Check sheet for the modelled part. Datum: model origin and axes. Units: mm. Face numbers are marked on the shaded views. A direction names the side the tool comes from. Round coordinates to 2 decimals unless told otherwise and drop trailing zeros. Write each loop counter-clockwise with the first axis right and the second up, starting at its lowest first coordinate (ties: lowest second). Pieces come first, ordered by that corner, then holes.
Item 1: Cross-section at A-A on y = -9.5. Enter the section's corners in (x, z), plus the area to 3 significant figures.
Item 2: Material ranges on line 1 (Z direction, x = -2, y = -8); line 2 (X direction, y = -3, z = 1); line 3 (Y direction, x = -6, z = 2.25), recorded low to high.
Item 3: Go/stop test with flat-tipped pins: pin 1 Ø3 at (x, y) = (0, -7) entering from +Z; pin 2 Ø1.2 at (y, z) = (-18.5, 0.5) entering from +X; pin 3 Ø2 at (y, z) = (13, 1.5) entering from -X. Record where each tip stops, or that it passes through.
Item 4: Tool access check on the marked faces 1, 2 and 3. Record the directions out of +Z, -Z, +X, -X, +Y, -Y that give a thin tool (end or side, any length) a straight path to the whole face; none if there is none.
from build123d import *

# Parameters (mm, degrees)
F1_DEPTH = 5
F2_R     = 4.999
F4_DEPTH = 1.25


# Not quite as in the source:
# - a fillet or chamfer is up to 0.001 mm smaller than in the source, because OpenCascade refuses the exact size


with BuildPart() as f1:
    # F0 (on Top) → F1 (new body, symmetric)
    with BuildSketch(Plane.XY):
        with BuildLine():
            add(Edge.make_bspline(
                [(-13.7097453699, 0), (-14.7537661126, 14.3834786699), (-16.3965507437, 37.0161302377), (-10.0715641044, 50.9942741703), (-3.1640643241, 51.6181998618), (0, 51.9039966166)],
                knots=[0, 0, 0, 0, 0.4858446106, 0.7644848677, 1, 1, 1, 1], degree=3))
            Line((-13.7097453699, 0), (13.7097453699, 0))
            add(Edge.make_bspline(
                [(13.7097453699, 0), (14.7537661126, 14.3834786699), (16.3965507437, 37.0161302377), (10.0715641044, 50.9942741703), (3.1640643241, 51.6181998618), (0, 51.9039966166)],
                knots=[0, 0, 0, 0, 0.4858446106, 0.7644848677, 1, 1, 1, 1], degree=3))
        make_face()
    extrude(amount=F1_DEPTH, both=True)

    # F2 (radius 5 in the source; OpenCascade refuses exactly that, so slightly less here)
    f2_edges = [f1.edges().sort_by_distance(p)[0] for p in [
        (-14.960078, 30.185645, 5),
        (14.960078, 30.185645, 5),
        (-14.960078, 30.185645, -5),
        (14.960078, 30.185645, -5),
    ]]
    fillet(f2_edges, radius=F2_R)

    # F3 (on Top) → F4 (join, symmetric)
    with BuildSketch(Plane.XY):
        Polygon((3.1797995325, 15.8989857882), (0, 15.8989857882), (-3.1797995325, 15.8989857882), (-3.1797995325, -33.4308445454), (0, -33.4308445454), (3.1797995325, -33.4308445454), align=None)
    extrude(amount=F4_DEPTH, both=True)


solid = f1.part
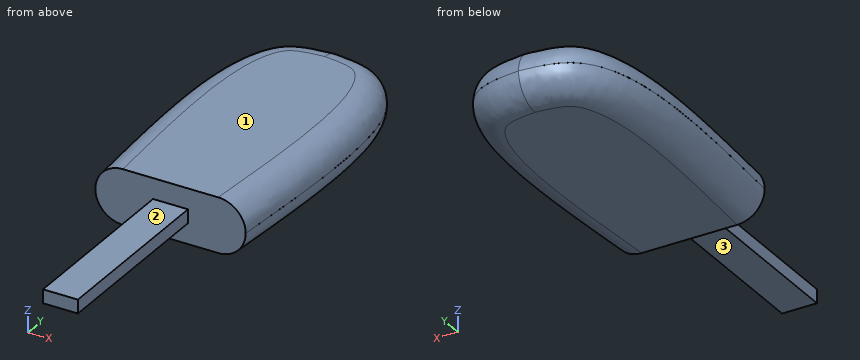
Response values:
1. outline: (-3.18, -1.25) - (3.18, -1.25) - (3.18, 1.25) - (-3.18, 1.25) - close
1. area: 15.9 mm2
2. line 1: z = -1.25 to 1.25
2. line 2: x = -3.18 to 3.18
2. line 3: y = 0 to 50.4
3. pin 1: stops at z = 1.25
3. pin 2: stops at x = 3.18
3. pin 3: stops at x = -14.58
4. face 1: +Z, +X, -X, +Y, -Y
4. face 2: +Z, +X, -X, -Y
4. face 3: -Z, +X, -X, -Y
